from build123d import *

# Parameters (mm, degrees)
SKETCH1_R           = 6
BOSS_EXTRUDE1_DEPTH = 33.65
FILLET2_R           = 5
SHELL1_OUTLINE_R    = 5
SHELL1_DEPTH        = 23.65
SCALE1_SCALE        = 2


# Read off the part's stored shape, not the designer's step: Shell1
with BuildPart() as part:
    # Sketch1 → Boss-Extrude1 (new body)
    with BuildSketch(Plane(origin=(0, 0, 0), x_dir=(1, 0, 0), z_dir=(0, 1, 0))):
        with Locations(Location((0, 0, 0), (0, 0, 270))):
            Circle(SKETCH1_R)
    extrude(amount=BOSS_EXTRUDE1_DEPTH)

    # Fillet2
    fillet2_edges = [part.edges().sort_by_distance(p)[0] for p in [
        (0, 33.65, -6),
    ]]
    fillet(fillet2_edges, radius=FILLET2_R)

    # Shell1 outline → Shell1 (cut)
    with BuildSketch(Plane(origin=(0, 0, 0), x_dir=(1, 0, 0), z_dir=(0, 1, 0))):
        Circle(SHELL1_OUTLINE_R)
    extrude(amount=SHELL1_DEPTH, mode=Mode.SUBTRACT)


with BuildPart() as part_1:
    # Scale1: scaled about (0, 20.592026778, 0)
    add(part.part.scale(SCALE1_SCALE).moved(Location((0, -20.592026778, 0))))


solid = part_1.part
Work out the finished part from the listing and answer in its coordinate system (mm). A direction names the side the tool comes from. Give positions to 0.01 mm unless a question says otherwise; leave off trailing zeros. Loops run counter-clockwise (first coordinate to the right, second up) from the corner with the lowest first, then second, coordinate; pieces in that order, holes last. Notation, with made-up numbers: (36, -12.75) - (82, -12.75) arc R21 cw to (82, -5.75) - close; hole circle Ø2 at (-30.5, 86). An arc over 180 degrees is marked (long way). Answer in a Markdown table with one row per item. Add a question column.
Q1. Consider line 1 along X through (y, z) = (0, 0); line 2 along Y through (x, z) = (0.25, 1.5); line 3 along X through (y, z) = (-17, -8.5). Determine where each line is inside the solid, lowest interval first.
Q2. Each of these flat-tipped pins is pushed along its axis until it touches: P1, Ø2, axis at y = -10.5, z = -4.5, coming from the +X side; P2, Ø10, axis at x = -8, y = 13.5, coming from the +Z side; P3, Ø6, axis at x = -0.5, z = -9, coming from the +Y side. Where does it stop, or does it pass through?
Q3. A tool of negligible diameter and unlimited length cuts with its end or side. For faces 4 (the cylindrical face through (-2.17, 2.73, 9.76)), 5 (the flat face through (9, -20.592, -5)), from which of +Z, -Z, +X, -X, +Y, -Y can it reach the whole face along a straight path? Write none if from no direction.
Q4. The part is cut by section A-A (y = 2.5). Determine the outline of the cut face in (x, z).
Q5. Determine the mould class of faces 1 (the flat face through (0, 46.708, 0)), 2 (the cylindrical face through (3.604, 7.657, 11.446)), 3 (the flat face through (0, 26.708, 0)) for opening direction Z: released by +Z, released by -Z, zero draft, split by the parting line, or undercut.
Solution:
| question | item | result |
|---|---|---|
| 1 | line 1 | x = -12 to -10, 10 to 12 |
| 1 | line 2 | y = 26.71 to 46.71 |
| 1 | line 3 | x = -8.47 to -5.27, 5.27 to 8.47 |
| 2 | P1 | stops at x = 11.48 |
| 2 | P2 | stops at z = 11.62 |
| 2 | P3 | stops at y = 45.87 |
| 3 | face 4 | -Y |
| 3 | face 5 | +Z, -Z, +X, -X, -Y |
| 4 | outline | circle Ø24 at (0, 0); hole circle Ø20 at (0, 0) |
| 5 | face 1 | zero draft |
| 5 | face 2 | split by the parting line |
| 5 | face 3 | undercut |
